from build123d import *

# Parameters (mm, degrees)
FILLET1_R   = 0.2
HEX_START   = -2.3
HEX_2_DEPTH = 2.3


with BuildPart() as part:
    # BodySke → BaseBody (revolve)
    with BuildSketch(Plane.XY, mode=Mode.PRIVATE) as basebody_sk:
        Polygon((0, 0), (0, 4.82), (0.48, 4.82), (2.8, 2.5), (24.555, 2.5), (25, 2.055), (25, 0), align=None)
    revolve(basebody_sk.sketch.rotate(Axis((0, 0, 0), (1, 0, 0)), 90), axis=Axis((0, 0, 0), (1, 0, 0)))

    # Fillet1
    fillet1_edges = [part.edges().sort_by_distance(p)[0] for p in [
        (2.8, 0, -2.5),
    ]]
    fillet(fillet1_edges, radius=FILLET1_R)

    # Hex 2: read off the stored shape, not the designer's step
    # Hex 2 outline → Hex 2 (cut)
    with BuildSketch(Plane.ZY.offset(HEX_START)):
        Polygon((-1.51, -0.871798906), (0, -1.743597813), (1.51, -0.871798906), (1.51, 0.871798906), (0, 1.743597813), (-1.51, 0.871798906), align=None)
    extrude(amount=HEX_2_DEPTH, mode=Mode.SUBTRACT)

    # Hex 2 2 outline → Hex 2 2 (revolve, cut)
    with BuildSketch(Plane.YX):
        Polygon((1.51, 2.3), (0, 3.171798906), (0, 2.3), align=None)
    revolve(axis=Axis((0, 0, 0), (1, 0, 0)), mode=Mode.SUBTRACT)


solid = part.part
Could you check a few things on this model? Use its own coordinates, in mm. A direction names the side the tool comes from. Give positions to 0.01 mm unless a question says otherwise; leave off trailing zeros. Order: outer loops, then holes, each group sorted by start corner. A loop starts at its lowest first (then second) coordinate and runs counter-clockwise, first axis right, second up.
1. Which directions (+Z, -Z, +X, -X, +Y, -Y) give clear straight access to the entire face, cutting with the end or side of a thin tool? Please do faces 4 (the cylindrical face through (0.243, 4.705, -1.045)), 5 (the flat face through (1.166, -1.314, 0.744)), 6 (the cylindrical face through (13.871, -0.751, 2.385)).
Answers below:
face 4: +X, -X
face 5: -X
face 6: +X
2. For pin 1 (1.9 mm diameter, centred on x = 1.5, y = 0, fed in from +Z), with a flat end and sliding along its axis, tell me the tip position at first contact or that it passes through.
Answers below:
pin 1: stops at z = 4.75
3. Suppose I cut it at A-A (x = 13.5). Write out the boundary of the cut face in (y, z), plus the area to 3 significant figures.
Answers below:
outline: circle Ø5 at (0, 0)
area: 19.6 mm2
4. Thinking about a two-plate mould opening in Y: for faces 1 (the flat face through (1, 0, 1.51)), 2 (the conical face through (2.63, 2.37, 1.23)), 3 (the flat face through (0, 2, 0)), which applies, +Y half, -Y half, draft (parallel to the pull), parting line (faces both ways), or undercut?
Answers below:
face 1: undercut
face 2: parting line
face 3: draft
5. I need wall thicknesses on L1, parallel to Y at x = 12.5, z = 1.75; L2, parallel to Y at x = 3, z = -2. Which ranges of each line are inside material? Lowest first, please.
Answers below:
L1: y = -1.79 to 1.79
L2: y = -1.5 to 1.5
